Geometry: see drawing. Coordinates: mm, zero at the bounding-box minimum. A direction names the side the tool comes from. Give positions to 0.01 mm unless a question says otherwise; leave off trailing zeros. Loops run counter-clockwise (first coordinate to the right, second up) from the corner with the lowest first, then second, coordinate; pieces in that order, holes last. Notation, with made-up numbers: (-20.75, -25) -> (36.25, -25) arc R19 ccw to (36.25, 10) -> close; hole circle Ø2 at (-5, -1.75). An arc over 180 degrees is marked (long way). Use CSV: the item, a comma, the result in double quotes.
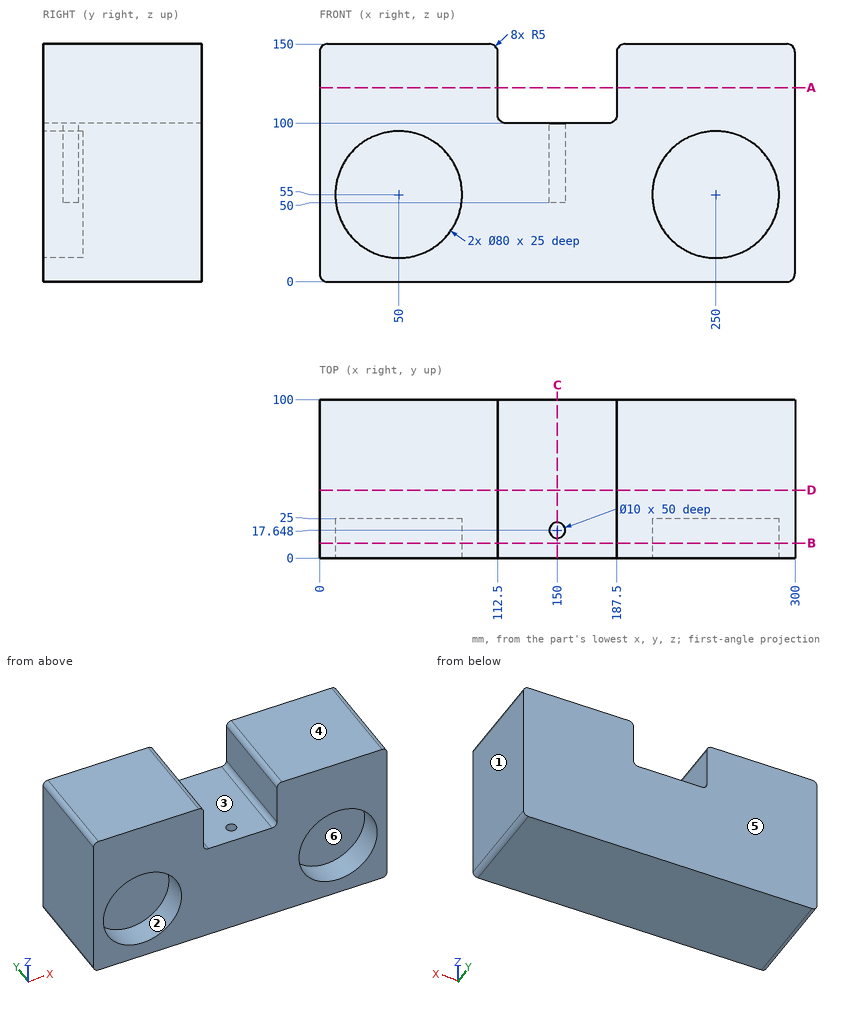
1) Section query A-A (z = 122.5). Return loops of the section in (x, y).
From the geometry:
outline,"(0, 0) -> (112.5, 0) -> (112.5, 100) -> (0, 100) -> close; (187.5, 0) -> (300, 0) -> (300, 100) -> (187.5, 100) -> close"
2) Section query D-D (y = 43). Return loops of the section in (x, z).
From the geometry:
outline,"(0, 5) arc R5 ccw to (5, 0) -> (295, 0) arc R5 ccw to (300, 5) -> (300, 145) arc R5 ccw to (295, 150) -> (192.5, 150) arc R5 ccw to (187.5, 145) -> (187.5, 105) arc R5 cw to (182.5, 100) -> (117.5, 100) arc R5 cw to (112.5, 105) -> (112.5, 145) arc R5 ccw to (107.5, 150) -> (5, 150) arc R5 ccw to (0, 145) -> close"
3) Reachability of the marked faces 1, 2 and 3 from +Z, -Z, +X, -X, +Y, -Y: full face, straight path, thin tool, end or side. Return the list, or none.
From the geometry:
face 1,"+Z, -Z, +X, +Y, -Y"
face 2,"-Y"
face 3,"+Z, +Y, -Y"
4) Section query B-B (y = 9.5). Return loops of the section in (x, z), then the cut area to 3 significant figures.
From the geometry:
outline,"(0, 5) arc R5 ccw to (5, 0) -> (295, 0) arc R5 ccw to (300, 5) -> (300, 145) arc R5 ccw to (295, 150) -> (192.5, 150) arc R5 ccw to (187.5, 145) -> (187.5, 105) arc R5 cw to (182.5, 100) -> (117.5, 100) arc R5 cw to (112.5, 105) -> (112.5, 145) arc R5 ccw to (107.5, 150) -> (5, 150) arc R5 ccw to (0, 145) -> close; hole circle Ø80 at (50, 55); hole circle Ø80 at (250, 55)"
area,"31,200 mm^2"
5) Section query C-C (x = 150). Return loops of the section in (y, z), then the cut area to 3 significant figures.
From the geometry:
outline,"(0, 0) -> (100, 0) -> (100, 100) -> (22.65, 100) -> (22.65, 50) -> (12.65, 50) -> (12.65, 100) -> (0, 100) -> close"
area,"9,500 mm^2"
6) Contact query for flat-ended pins moving along their axis: pin 1 (8 mm diameter, centred on x = 149.5, y = 20, fed in from +Z); pin 2 (6 mm diameter, centred on x = 239.5, z = 26.5, fed in from -Y). Output: stop coordinate, or through.
From the geometry:
pin 1,"stops at z = 100"
pin 2,"stops at y = 25"
7) Ray query, line 1 (X direction, y = 48, z = 111.5); line 2 (Z direction, x = 250, y = 17.75); line 3 (Y direction, x = 30.5, z = 35.5). Return the intervals inside material, ascending.
From the geometry:
line 1,"x = 0 to 112.5, 187.5 to 300"
line 2,"z = 0 to 15, 95 to 150"
line 3,"y = 25 to 100"
8) Mould query, pull axis Z, two halves, no side actions, for the marked faces 4, 5 and 6. Classes: pulls with the +Z half, pulls with the -Z half, needs draft (parallel to the pull), parting line crosses it, or undercut.
From the geometry:
face 4,"pulls with the +Z half"
face 5,"needs draft"
face 6,"undercut"
